Job drawing, mm, ordinate dimensions from the low corner. One solid piece. Coordinates: 2 decimals unless noted, no trailing zeros. Write each loop counter-clockwise with the first axis right and the second up, starting at its lowest first coordinate (ties: lowest second). Pieces come first, ordered by that corner, then holes. Notation, with made-up numbers: (17.25, 83.5) - (75.25, 83.5) arc R30 cw to (75.25, 105.5) - close; hole circle Ø11 at (-13.5, -37). An arc over 180 degrees is marked (long way). Put each result on its own line as item: value. Start each with the question number.
1. Saw through at A-A, the plane z = 28.5. Write the cut outline in (x, y), plus the area to 3 significant figures.
2. Saw through at C-C, the plane y = 0.65. Write the cut outline in (x, z), plus the area to 3 significant figures.
3. Drop flat-ended pins along their axis: P1, Ø4, axis at x = 28.5, z = 53.3, coming from the +Y side; P2, Ø21, axis at x = 27, z = 24.5, coming from the +Y side; P3, Ø2, axis at x = 31.5, y = 3, coming from the +Z side. Give the stop position or say it passes through.
4. Saw through at D-D, the plane z = 53.3. Write the cut outline in (x, y), plus the area to 3 significant figures.
5. Saw through at B-B, the plane x = 28.5. Write the cut outline in (y, z), plus the area to 3 significant figures.
6. Drill centre lines: L1, parallel to X at y = 1.4, z = 28.5; L2, parallel to X at y = 3.6, z = 28.5; L3, parallel to X at y = 2.95, z = 39.5. Where is each one in solid material? Low to high. Write a range as from..to.
7. Pull direction X, two halves, no side cores. Call the marked faces 1, 2 and 3: released by +X, released by -X, zero draft, split by the parting line, or undercut.
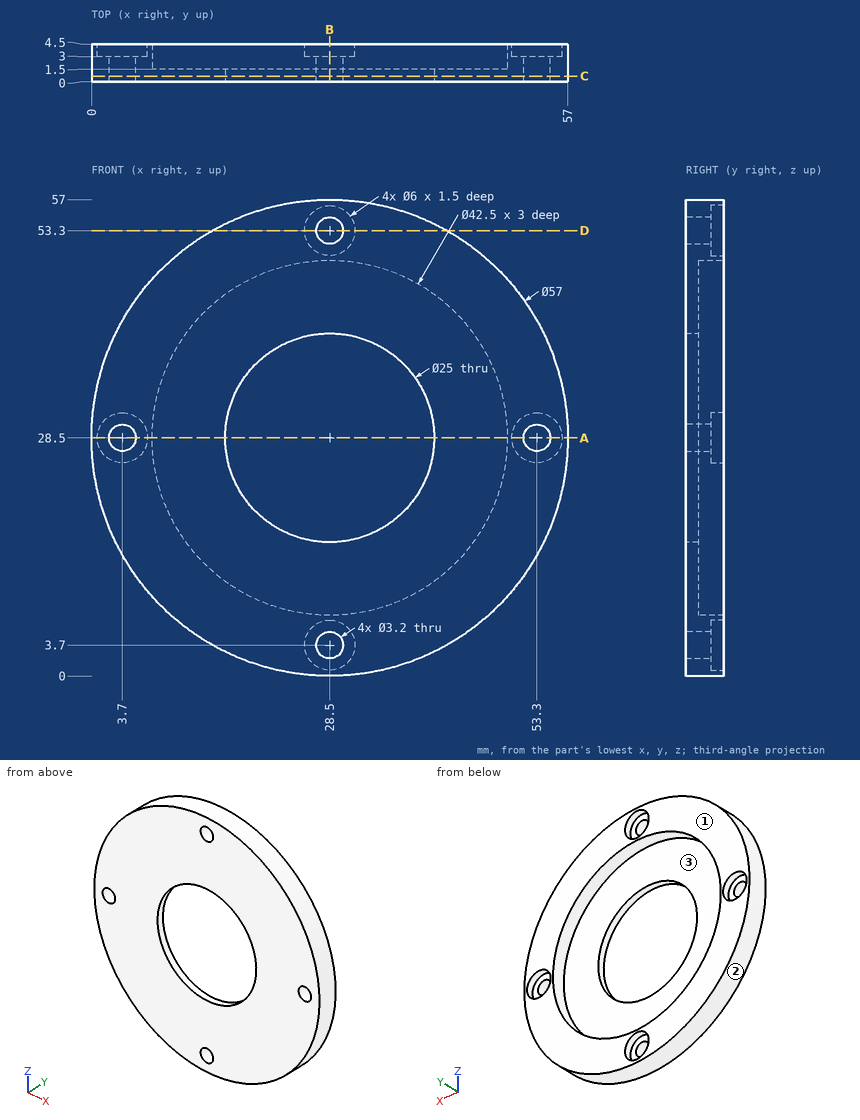
Final values:
1. outline: (0, 0) - (2.1, 0) - (2.1, 3) - (0.7, 3) - (0.7, 4.5) - (0, 4.5) - close; (5.3, 0) - (16, 0) - (16, 1.5) - (7.25, 1.5) - (7.25, 4.5) - (6.7, 4.5) - (6.7, 3) - (5.3, 3) - close; (41, 0) - (51.7, 0) - (51.7, 3) - (50.3, 3) - (50.3, 4.5) - (49.75, 4.5) - (49.75, 1.5) - (41, 1.5) - close; (54.9, 0) - (57, 0) - (57, 4.5) - (56.3, 4.5) - (56.3, 3) - (54.9, 3) - close
1. area: 54.3 mm²
2. outline: circle Ø57 at (28.5, 28.5); hole circle Ø3.2 at (3.7, 28.5); hole circle Ø25 at (28.5, 28.5); hole circle Ø3.2 at (28.5, 3.7); hole circle Ø3.2 at (28.5, 53.3); hole circle Ø3.2 at (53.3, 28.5)
2. area: 2,030 mm²
3. P1: stops at y = 3
3. P2: stops at y = 1.5
3. P3: stops at z = 56.93
4. outline: (14.46, 0) - (26.9, 0) - (26.9, 3) - (25.5, 3) - (25.5, 4.5) - (14.46, 4.5) - close; (30.1, 0) - (42.54, 0) - (42.54, 4.5) - (31.5, 4.5) - (31.5, 3) - (30.1, 3) - close
4. area: 108 mm²
5. outline: (0, 0) - (4.5, 0) - (4.5, 0.7) - (3, 0.7) - (3, 2.1) - (0, 2.1) - close; (0, 5.3) - (3, 5.3) - (3, 6.7) - (4.5, 6.7) - (4.5, 7.25) - (1.5, 7.25) - (1.5, 16) - (0, 16) - close; (0, 41) - (1.5, 41) - (1.5, 49.75) - (4.5, 49.75) - (4.5, 50.3) - (3, 50.3) - (3, 51.7) - (0, 51.7) - close; (0, 54.9) - (3, 54.9) - (3, 56.3) - (4.5, 56.3) - (4.5, 57) - (0, 57) - close
5. area: 54.3 mm²
6. L1: x = 0..2.1, 5.3..16, 41..51.7, 54.9..57
6. L2: x = 0..0.7, 6.7..7.25, 49.75..50.3, 56.3..57
6. L3: x = 2.21..10.32, 46.68..54.79
7. face 1: zero draft
7. face 2: split by the parting line
7. face 3: undercut
